The listing builds one solid part. Answer for the finished solid, in the listing's coordinates (mm). A direction names the side the tool comes from. Round coordinates to 2 decimals unless told otherwise and drop trailing zeros. Write each loop counter-clockwise with the first axis right and the second up, starting at its lowest first coordinate (ties: lowest second). Pieces come first, ordered by that corner, then holes.
from build123d import *

# Parameters (mm, degrees)
CHAMFER_2_SIZE           = 1
CHAMFER_1_SIZE           = 1
CUT_EXTRUDE_1_DEPTH      = 140.773030303
CUT_EXTRUDE_1_DEPTH_BACK = 140.773030303
SKETCH_2_W               = 45.54274113
SKETCH_2_H               = 12
SKETCH_3_OUTSIDE_W       = 99.17
SKETCH_3_OUTSIDE_H       = 99.17
SKETCH_3_OUTSIDE_W_2     = 70.7839493
SKETCH_3_OUTSIDE_H_2     = 28
CUT_EXTRUDE_1_2_DEPTH    = 38
FILLET_1_R               = 5
SKETCH_4_R               = 6.5
CUT_EXTRUDE_2_DEPTH      = 38


# Read off the part's stored shape, not the designer's step: M4 螺纹孔1
with BuildPart() as part:
    # 草图1 → 旋转1 (revolve)
    with BuildSketch(Plane.XY, mode=Mode.PRIVATE) as revolve_1_sk:
        Polygon((0, 0), (0, 32.5), (2.8, 32.5), (2.8, 27.5), (9, 27.5), (9, 32.5), (12.4, 32.5), (12.4, 27.5), (18.6, 27.5), (18.6, 32.5), (22, 32.5), (22, 15), (25, 15), (25, 16), (132, 16), (132, 0), align=None)
    revolve(revolve_1_sk.sketch.rotate(Axis((0, 0, 0), (1, 0, 0)), 90), axis=Axis((0, 0, 0), (1, 0, 0)))

    # 倒角2
    chamfer_2_edges = [part.edges().sort_by_distance(p)[0] for p in [
        (132, 0, -16),
    ]]
    chamfer(chamfer_2_edges, length=CHAMFER_2_SIZE)

    # 倒角1
    chamfer_1_edges = [part.edges().sort_by_distance(p)[0] for p in [
        (0, 0, -32.5),
    ]]
    chamfer(chamfer_1_edges, length=CHAMFER_1_SIZE)

    # 草图2 → Cut-Extrude 1 (cut, two sides: drawn at the far end of the back side and taken through both)
    with BuildSketch(Plane.XY.offset(-CUT_EXTRUDE_1_DEPTH_BACK)):
        with Locations((112.771370565, 0)):
            Rectangle(SKETCH_2_W, SKETCH_2_H)
    extrude(amount=CUT_EXTRUDE_1_DEPTH + CUT_EXTRUDE_1_DEPTH_BACK, mode=Mode.SUBTRACT)

    # 草图3 outside → Cut-Extrude 1 2 (cut)
    with BuildSketch(Plane(origin=(132, 0, 0), x_dir=(0, 0, -1), z_dir=(1, 0, 0))):
        Rectangle(SKETCH_3_OUTSIDE_W, SKETCH_3_OUTSIDE_H)
        Rectangle(SKETCH_3_OUTSIDE_W_2, SKETCH_3_OUTSIDE_H_2, mode=Mode.SUBTRACT)
    extrude(amount=-CUT_EXTRUDE_1_2_DEPTH, mode=Mode.SUBTRACT)

    # 圆角1
    # the kernel refuses this fillet: 5 mm, written as the material it adds along each edge
    with BuildSketch(Plane(origin=(94, -14, 20.245966692), x_dir=(1, 0, 0), z_dir=(0, 0, -1))) as fillet_1_piece_1_section:
        with BuildLine():
            CenterArc((FILLET_1_R, FILLET_1_R), FILLET_1_R, 180, 90)
            Line((0, FILLET_1_R), (0, 0))
            Line((0, 0), (FILLET_1_R, 0))
        make_face()
    fillet_1_piece_1 = extrude(amount=40.491933385, mode=Mode.PRIVATE)
    fillet_1_piece_1 = fillet_1_piece_1 & Plane(origin=(95.499656212, 0, 0), x_dir=(0, 0, 1), z_dir=(1, 0, 0)) * Cylinder(16, 101, mode=Mode.PRIVATE)
    add(fillet_1_piece_1)
    with BuildSketch(Plane(origin=(94, 14, -20.245966692), x_dir=(1, 0, 0), z_dir=(0, 0, 1))) as fillet_1_piece_2_section:
        with BuildLine():
            CenterArc((FILLET_1_R, FILLET_1_R), FILLET_1_R, 180, 90)
            Line((0, FILLET_1_R), (0, 0))
            Line((0, 0), (FILLET_1_R, 0))
        make_face()
    fillet_1_piece_2 = extrude(amount=40.491933385, mode=Mode.PRIVATE)
    fillet_1_piece_2 = fillet_1_piece_2 & Plane(origin=(95.499656212, 0, 0), x_dir=(0, 0, 1), z_dir=(1, 0, 0)) * Cylinder(16, 101, mode=Mode.PRIVATE)
    add(fillet_1_piece_2)

    # 草图4 → 切除-拉伸2 (cut)
    with BuildSketch(Plane(origin=(0, 14, 0), x_dir=(1, 0, 0), z_dir=(0, 1, 0))):
        with Locations(Location((114, 0, 0), (0, 0, 180))):
            Circle(SKETCH_4_R)
    extrude(amount=-CUT_EXTRUDE_2_DEPTH, mode=Mode.SUBTRACT)

    # M4 螺纹孔1 outline → M4 螺纹孔1 (revolve, cut)
    with BuildSketch(Plane(origin=(0, 10, 0), x_dir=(0, 1, 0), z_dir=(0, 0, -1))):
        Polygon((0, 120.286969782), (1.65, 120.286969782), (1.65, 131.625), (2.025, 132), (0, 132), align=None)
    revolve(axis=Axis((0, 10, 0), (1, 0, 0)), mode=Mode.SUBTRACT)


solid = part.part
1. Straight lines are drawn through the part: line 1 along X through (y, z) = (-13, -25); line 2 along Y through (x, z) = (124, 0); line 3 along Y through (x, z) = (96, -6). For each, find the intervals that lie inside material, in ascending order.
Geometry says:
line 1: x = 0 to 2.8, 9 to 12.4, 18.6 to 22
line 2: y = -14 to -6, 6 to 8.35, 11.65 to 14
line 3: y = -14.83 to -6, 6 to 14.83
2. For a pull along Z with two mould halves and no side action, classify faces 4 (the face through (22, 7, 14)), 5 (the face through (10.72, -9.76, 31)), 6 (the face through (126.035, 11.524, -0.632)) as released by +Z, released by -Z, zero draft, split by the parting line, or undercut.
Geometry says:
face 4: zero draft
face 5: split by the parting line
face 6: undercut
3. Section C-C on z = 0 is taken. Give the number of separate pieces and of enclosed holes in the cut face, plus the area to 3 significant figures.
Geometry says:
separate pieces: 4
enclosed holes: 0
area: 3,930 mm2
4. Section D-D on x = 72 is taken. Determine the outline of the cut face in (y, z).
Geometry says:
outline: circle Ø32 at (0, 0)
5. A tool of negligible diameter and unlimited length cuts with its end or side. For faces 1 (the face through (90, 0, 0)), 2 (the face through (15.543, 24.397, 12.69)), 3 (the face through (97.21, 14.33, -0.11)), from which of +Z, -Z, +X, -X, +Y, -Y can it reach the whole face along a straight path? Write none if from no direction.
Geometry says:
face 1: +Z, -Z, +X
face 2: none
face 3: +Z, -Z, +X, +Y
6. Given pin 1 (4.5 mm diameter, centred on y = 10, z = 0, fed in from -X); pin 2 (17 mm diameter, centred on x = 120, z = -2, fed in from -Y); pin 3 (10 mm diameter, centred on x = 73.5, y = 15, fed in from +Z); pin 4 (12.5 mm diameter, centred on x = 112.5, z = -1, fed in from +Y), each flat-ended and moving along its own axis, determine where each tip first touches the part or whether it passes through.
Geometry says:
pin 1: stops at x = 0
pin 2: stops at y = -14
pin 3: stops at z = 12.49
pin 4: stops at y = 14
7. Section B-B on x = 114 is taken. Determine the outline of the cut face in (y, z).
Geometry says:
outline: (-14, -7.75) arc R16 ccw to (-6, -14.83) - (-6, -6.5) - (-14, -6.5) - close; (-14, 6.5) - (-6, 6.5) - (-6, 14.83) arc R16 ccw to (-14, 7.75) - close; (6, -14.83) arc R16 ccw to (14, -7.75) - (14, -6.5) - (6, -6.5) - close; (6, 6.5) - (14, 6.5) - (14, 7.75) arc R16 ccw to (6, 14.83) - close
